from build123d import *

# Parameters (mm, degrees)
BOSS_EXTRUDE1_DEPTH = 34.925
CUT_EXTRUDE1_DEPTH  = 40.820120417
LPATTERN1_COUNT     = 2
LPATTERN1_PITCH     = 25
LPATTERN1_COL_COUNT = 2
LPATTERN1_COL_PITCH = 25


with BuildPart() as part:
    # Sketch1 → Boss-Extrude1 (new, symmetric)
    with BuildSketch(Plane(origin=(0, 0, 0), x_dir=(1, 0, 0), z_dir=(0, 1, 0))):
        Polygon((-15.875, 0), (0, 0), (0, 1.4478), (-12.6365, 1.4478), (-12.6365, 7.366), (-17.653, 7.366), (-17.653, 6.477), (-13.5255, 6.477), (-13.5255, 2.286), align=None)
        Polygon((0, 1.4478), (0, 0), (15.875, 0), (13.5255, 2.286), (13.5255, 6.477), (17.653, 6.477), (17.653, 7.366), (12.6365, 7.366), (12.6365, 1.4478), align=None)
    extrude(amount=BOSS_EXTRUDE1_DEPTH, both=True)

    # Sketch2 → Cut-Extrude1 (cut, through all)
    with BuildSketch(Plane.XY):
        with BuildLine():
            Line((-2.667, -4.833), (-2.667, 4.833))
            ThreePointArc((-2.667, 4.833), (0, 7.5), (2.667, 4.833))
            Line((2.667, 4.833), (2.667, -4.833))
            ThreePointArc((2.667, -4.833), (0, -7.5), (-2.667, -4.833))
        make_face()
    cut_extrude1 = extrude(amount=-CUT_EXTRUDE1_DEPTH, mode=Mode.SUBTRACT)

    # LPattern1: Cut-Extrude1 ×2
    with Locations(*[(0, -i * LPATTERN1_PITCH, 0) for i in range(1, LPATTERN1_COUNT)]):
        add(cut_extrude1, mode=Mode.SUBTRACT)

    # LPattern1 col: Cut-Extrude1 ×2
    with Locations(*[(0, i * LPATTERN1_COL_PITCH, 0) for i in range(1, LPATTERN1_COL_COUNT)]):
        add(cut_extrude1, mode=Mode.SUBTRACT)


solid = part.part
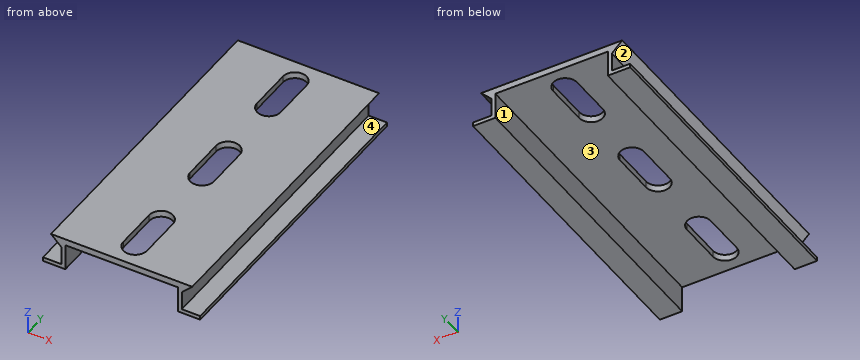
Here's how the part is built. I have some questions about the finished solid (model axes, mm). Face numbers are marked on the shaded views. Round coordinates to 2 decimals unless told otherwise and drop trailing zeros. Write each loop counter-clockwise with the first axis right and the second up, starting at its lowest first coordinate (ties: lowest second). Pieces come first, ordered by that corner, then holes. Notation, with made-up numbers: (88.5, 66.25) -> (131.5, 66.25) arc R7 cw to (131.5, 70.25) -> close; hole circle Ø10 at (74.5, -35.5). An arc over 180 degrees is marked (long way). One line per item, written item: value.
1) I'm going to push flat-ended pins straight in: pin 1 Ø1.2 at (y, z) = (26, -1) entering from +X; pin 2 Ø0.7 at (y, z) = (1, -0.5) entering from +X; pin 3 Ø1.2 at (y, z) = (-2.5, -0.5) entering from -X (3 decimals). Where does each tip first touch, or does it pass through?
Filled sheet:
pin 1: stops at x = 15.46
pin 2: stops at x = 15.72
pin 3: stops at x = -15.875
2) Suppose I cut it at C-C on x = 0. List the corners of the cut face in (y, z) for me (3 decimals).
Filled sheet:
outline: (-34.925, -1.448) -> (-32.5, -1.448) -> (-32.5, 0) -> (-34.925, 0) -> close; (-17.5, -1.448) -> (-7.5, -1.448) -> (-7.5, 0) -> (-17.5, 0) -> close; (7.5, -1.448) -> (17.5, -1.448) -> (17.5, 0) -> (7.5, 0) -> close; (32.5, -1.448) -> (34.925, -1.448) -> (34.925, 0) -> (32.5, 0) -> close
3) Suppose I cut it at A-A on z = -3.75. List the corners of the cut face in (x, y) for me (1 decimal).
Filled sheet:
outline: (-13.5, -34.9) -> (-12.6, -34.9) -> (-12.6, 34.9) -> (-13.5, 34.9) -> close; (12.6, -34.9) -> (13.5, -34.9) -> (13.5, 34.9) -> (12.6, 34.9) -> close
4) If I drill on line 1 (X direction, y = -18, z = -6.75); line 2 (X direction, y = 20.5, z = -4); line 3 (Y direction, x = -2, z = -1.25) (3 decimals), over which ranges is the centre line in solid material (lowest first)? Write a range as [from, to].
Filled sheet:
line 1: x = [-17.65, -12.64], [12.64, 17.65]
line 2: x = [-13.53, -12.64], [12.64, 13.53]
line 3: y = [-34.925, -31.597], [-18.403, -6.597], [6.597, 18.403], [31.597, 34.925]
5) Suppose I cut it at D-D on y = -12.5. List the corners of the cut face in (x, z) for me (1 decimal), plus the area to 3 significant figures.
Filled sheet:
outline: (-17.7, -7.4) -> (-12.6, -7.4) -> (-12.6, -1.4) -> (12.6, -1.4) -> (12.6, -7.4) -> (17.7, -7.4) -> (17.7, -6.5) -> (13.5, -6.5) -> (13.5, -2.3) -> (15.9, 0) -> (-15.9, 0) -> (-13.5, -2.3) -> (-13.5, -6.5) -> (-17.7, -6.5) -> close
area: 62.4 mm2
6) Suppose I cut it at B-B on y = -22. List the corners of the cut face in (x, z) for me (1 decimal), plus the area to 3 significant figures.
Filled sheet:
outline: (-17.7, -7.4) -> (-12.6, -7.4) -> (-12.6, -1.4) -> (-2.7, -1.4) -> (-2.7, 0) -> (-15.9, 0) -> (-13.5, -2.3) -> (-13.5, -6.5) -> (-17.7, -6.5) -> close; (2.7, -1.4) -> (12.6, -1.4) -> (12.6, -7.4) -> (17.7, -7.4) -> (17.7, -6.5) -> (13.5, -6.5) -> (13.5, -2.3) -> (15.9, 0) -> (2.7, 0) -> close
area: 54.7 mm2
7) We'd pull the mould along X, two halves only. Please class the marked faces 1, 2, 3 and 4: released by +X, released by -X, zero draft, split by the parting line, or undercut.
Filled sheet:
face 1: undercut
face 2: released by -X
face 3: undercut
face 4: zero draft
